from build123d import *

# Parameters (mm, degrees)
SKETCH010_W     = 91
SKETCH010_H     = 10
PAD004_DEPTH    = 10
SKETCH011_R     = 1.5
POCKET006_DEPTH = 5
SKETCH012_R     = 1.5
POCKET007_DEPTH = 5


with BuildPart() as part:
    # Sketch010 → Pad004 (new body)
    with BuildSketch(Plane.XY):
        Rectangle(SKETCH010_W, SKETCH010_H)
    extrude(amount=PAD004_DEPTH)

    # Sketch011 (on Face1 of Pad004) → Pocket006 (cut)
    with BuildSketch(Plane(origin=(-45.5, 0, 0), x_dir=(0, -1, 0), z_dir=(-1, 0, 0))):
        with Locations((0, 5)):
            Circle(SKETCH011_R)
    extrude(amount=-POCKET006_DEPTH, mode=Mode.SUBTRACT)

    # Sketch012 (on Face7 of Pocket006) → Pocket007 (cut)
    with BuildSketch(Plane.YZ.offset(45.5)):
        with Locations((0, 5)):
            Circle(SKETCH012_R)
    extrude(amount=-POCKET007_DEPTH, mode=Mode.SUBTRACT)


solid = part.part
Model file for the job. Use its own axes, mm. A direction names the side the tool comes from. Round coordinates to 2 decimals unless told otherwise and drop trailing zeros. Order: outer loops, then holes, each group sorted by start corner. A loop starts at its lowest first (then second) coordinate and runs counter-clockwise, first axis right, second up.
(1) Pull direction Z, two halves, no side cores. Call faces 4 (the face through (-1, 5, 5)), 5 (the face through (-1, 0, 10)), 6 (the face through (-1, 0, 0)), 7 (the face through (40.5, 0, 5)): released by +Z, released by -Z, zero draft, split by the parting line, or undercut.
(2) 3-axis set-ups, long thin cutter, end or side, ignore diameter. For faces 1 (the face through (43.04, -1.5, 5.07)), 2 (the face through (45.5, -1.2, 3.8)), 3 (the face through (-43.04, 1.5, 5.07)): which of +Z, -Z, +X, -X, +Y, -Y reach the whole face in a straight line?
(3) Drill centre lines: line 1 (Z direction, x = -42.65, y = 0); line 2 (Z direction, x = 41.5, y = -0.75); line 3 (X direction, y = 0, z = 6). Where is each one in solid material? Low to high.
(4) Band-saw the part on A-A (y = 0). List the corners of the cut face in (x, z), then the cut area to 3 significant figures.
Verdict:
1. face 4: zero draft
1. face 5: released by +Z
1. face 6: released by -Z
1. face 7: undercut
2. face 1: +X
2. face 2: +Z, -Z, +X, +Y, -Y
2. face 3: -X
3. line 1: z = 0 to 3.5, 6.5 to 10
3. line 2: z = 0 to 3.7, 6.3 to 10
3. line 3: x = -40.5 to 40.5
4. outline: (-45.5, 0) - (45.5, 0) - (45.5, 3.5) - (40.5, 3.5) - (40.5, 6.5) - (45.5, 6.5) - (45.5, 10) - (-45.5, 10) - (-45.5, 6.5) - (-40.5, 6.5) - (-40.5, 3.5) - (-45.5, 3.5) - close
4. area: 880 mm2
